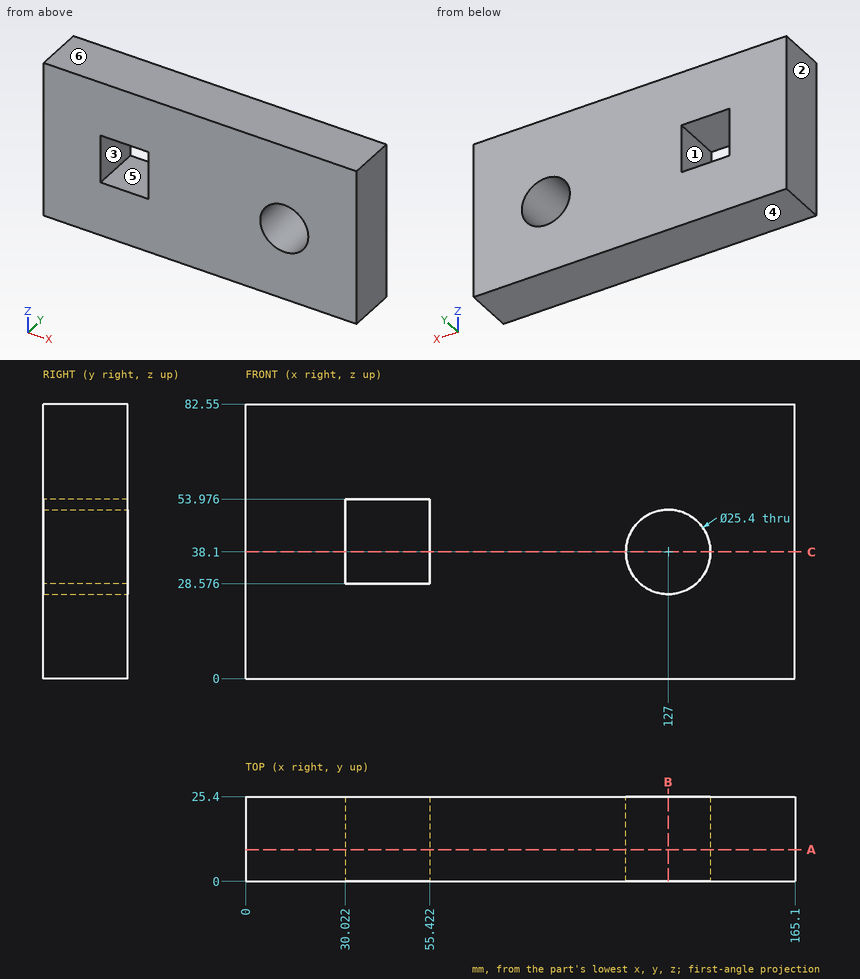
The drawing under review shows one solid part. Ordinate dimensions are in mm from its lowest x, y, z. A direction names the side the tool comes from. Give positions to 0.01 mm unless a question says otherwise; leave off trailing zeros. Write each loop counter-clockwise with the first axis right and the second up, starting at its lowest first coordinate (ties: lowest second). Pieces come first, ordered by that corner, then holes. Notation, with made-up numbers: M 42.5,-19.5 L 66.5,-19.5 A26 ccw 66.5,3.5 Z; hole C 74.25,13 d4. An arc over 180 degrees is marked long. Write each question's results on one line, items separated by ' | '. Start each with the question number.
1. We need section A-A (y = 9.5). Write out the cut boundary in (x, z), and give its area (3 significant figures).
2. We need section B-B (x = 127). Write out the cut boundary in (y, z).
3. We need section C-C (z = 38.1). Write out the cut boundary in (x, y).
4. For the marked faces 1 and 2, list the 3-axis set-ups (+Z, -Z, +X, -X, +Y, -Y) from which the entire face can be reached by the end or side of a thin tool; tool diameter is ignored.
5. Mouldability with a two-part tool opening along Z and no side actions: class the marked faces 3, 4, 5 and 6 as released by +Z, released by -Z, zero draft, split by the parting line, or undercut.
6. For probe 1 along X at (y, z) = (14, 38.1); probe 2 along Z at (x, y) = (37, 2.5); probe 3 along X at (y, z) = (12.25, 33), list the stretches that pass through material, from the lowest coordinate up. Write a range as [from, to].
Results found:
1) outline: M 0,0 L 165.1,0 L 165.1,82.55 L 0,82.55 Z; hole M 30.02,28.58 L 55.42,28.58 L 55.42,53.98 L 30.02,53.98 Z; hole C 127,38.1 d25.4 | area: 12,500 mm^2
2) outline: M 0,0 L 25.4,0 L 25.4,25.4 L 0,25.4 Z; M 0,50.8 L 25.4,50.8 L 25.4,82.55 L 0,82.55 Z
3) outline: M 0,0 L 30.02,0 L 30.02,25.4 L 0,25.4 Z; M 55.42,0 L 114.3,0 L 114.3,25.4 L 55.42,25.4 Z; M 139.7,0 L 165.1,0 L 165.1,25.4 L 139.7,25.4 Z
4) face 1: +Y, -Y | face 2: +Z, -Z, -X, +Y, -Y
5) face 3: undercut | face 4: released by -Z | face 5: undercut | face 6: released by +Z
6) probe 1: x = [0, 30.02], [55.42, 114.3], [139.7, 165.1] | probe 2: z = [0, 28.58], [53.98, 82.55] | probe 3: x = [0, 30.02], [55.42, 115.37], [138.63, 165.1]
